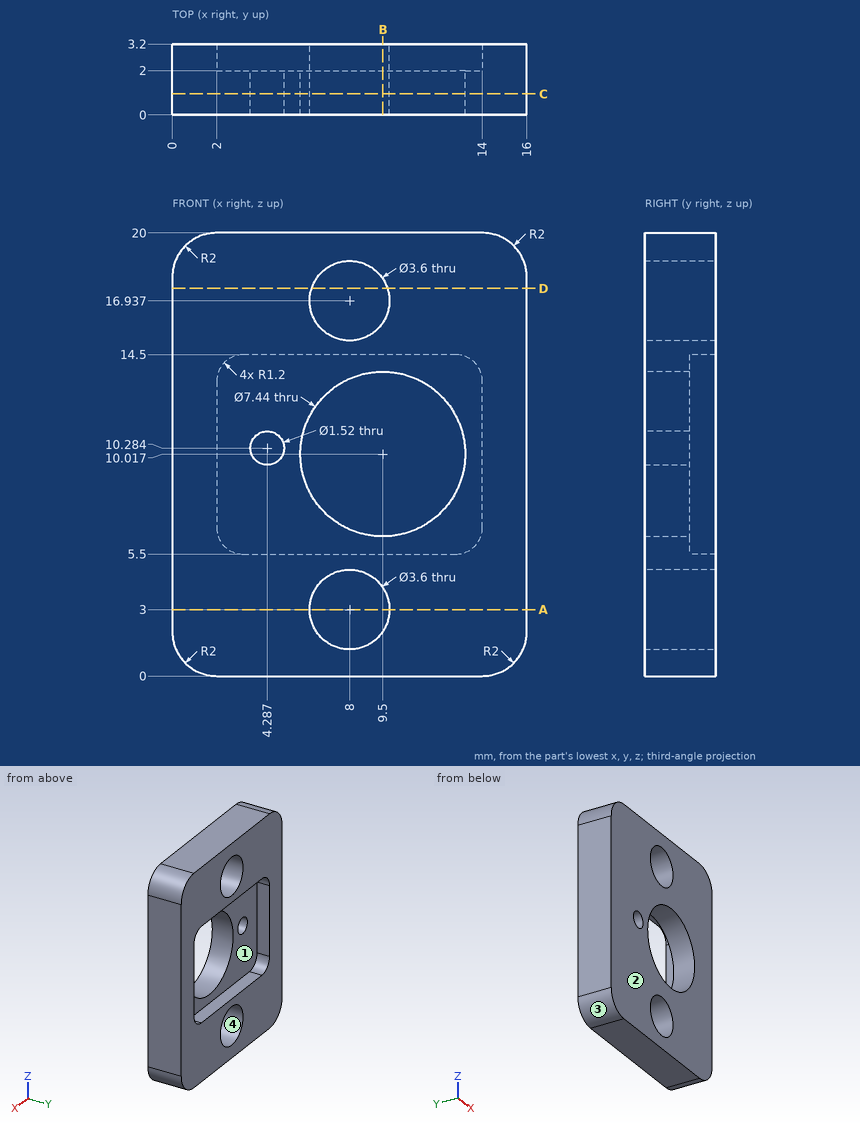
Job drawing, mm, ordinate dimensions from the low corner. One solid piece. Coordinates: 2 decimals unless noted, no trailing zeros. Order: outer loops, then holes, each group sorted by start corner. A loop starts at its lowest first (then second) coordinate and runs counter-clockwise, first axis right, second up. Notation, with made-up numbers: M 20,-22 L 44,-22 A24 ccw 44,-12 Z; hole C -2.5,58 d10. An arc over 180 degrees is marked long. One line per question, with ' | ' between items.
Q1. Slice it at A-A (z = 3). Give the cut face in (x, y).
A:
outline: M 0,0 L 6.2,0 L 6.2,3.2 L 0,3.2 Z; M 9.8,0 L 16,0 L 16,3.2 L 9.8,3.2 Z
Q2. Slice it at D-D (z = 17.5). Give the cut face in (x, y).
A:
outline: M 0,0 L 6.29,0 L 6.29,3.2 L 0,3.2 Z; M 9.71,0 L 16,0 L 16,3.2 L 9.71,3.2 Z
Q3. Two-plate mould, pull along X, no slides. Class the marked faces 1, 2, 3 and 4: +X half, -X half, draft (parallel to the pull), parting line (faces both ways), or undercut.
A:
face 1: undercut | face 2: draft | face 3: -X half | face 4: undercut
Q4. Drill centre lines: line 1 (Z direction, x = 4.25, y = 1.7) (1 decimal); line 2 (X direction, y = 0.75, z = 3); line 3 (Y direction, x = 12.25, z = 6.5). Where is each one in solid material? Low to high.
A:
line 1: z = 0 to 9.5, 11 to 20 | line 2: x = 0 to 6.2, 9.8 to 16 | line 3: y = 0 to 2
Q5. Pin check, flat tip, straight feed: P1, Ø4.5, axis at x = 9.5, z = 10.02, coming from the +Y side. Stop position of the tip, or through.
A:
P1: passes through
Q6. Slice it at C-C (y = 0.95). Give the cut face in (x, z).
A:
outline: M 0,2 A2 ccw 2,0 L 14,0 A2 ccw 16,2 L 16,18 A2 ccw 14,20 L 2,20 A2 ccw 0,18 Z; hole C 4.29,10.28 d1.52; hole C 9.5,10.02 d7.44; hole C 8,3 d3.6; hole C 8,16.94 d3.6
Q7. Slice it at B-B (x = 9.5). Give the cut face in (y, z) (1 decimal).
A:
outline: M 0,0 L 3.2,0 L 3.2,2 L 0,2 Z; M 0,4 L 3.2,4 L 3.2,5.5 L 2,5.5 L 2,6.3 L 0,6.3 Z; M 0,13.7 L 2,13.7 L 2,14.5 L 3.2,14.5 L 3.2,15.9 L 0,15.9 Z; M 0,17.9 L 3.2,17.9 L 3.2,20 L 0,20 Z
